Read the model definition and answer for the solid it produces. Units are mm, in the model's axes. A direction names the side the tool comes from. Coordinates: 2 decimals unless noted, no trailing zeros. Order: outer loops, then holes, each group sorted by start corner. A loop starts at its lowest first (then second) coordinate and runs counter-clockwise, first axis right, second up. Notation, with made-up numbers: (-28, 35) - (-9, 35) arc R16 ccw to (-9, 54) - close; hole circle Ø6 at (-34.75, 4). An arc over 180 degrees is marked (long way). Write item = value, one per line.
from build123d import *

# Parameters (mm, degrees)
SKETCH2_W                = 160
SKETCH2_H                = 130
BOSS_EXTRUDE1_DEPTH      = 6
SKETCH7_W                = 40
SKETCH7_H                = 40
CUT_EXTRUDE1_DEPTH       = 18
SKETCH9_R                = 2
CUT_EXTRUDE2_DEPTH       = 63
BOSS_EXTRUDE2_DEPTH      = 5
BOSS_EXTRUDE2_DEPTH_BACK = 10
SKETCH11_W               = 20
SKETCH11_H               = 15
CUT_EXTRUDE4_DEPTH       = 6
SKETCH13_R               = 2
CUT_EXTRUDE5_DEPTH       = 222
FILLET4_R                = 2
FILLET5_R                = 2
FILLET6_R                = 2


with BuildPart() as part:
    # Sketch2 → Boss-Extrude1 (new body)
    with BuildSketch(Plane(origin=(0, 0, 0), x_dir=(1, 0, 0), z_dir=(0, 1, 0))):
        Rectangle(SKETCH2_W, SKETCH2_H)
    extrude(amount=BOSS_EXTRUDE1_DEPTH)

    # Sketch7 → Cut-Extrude1 (cut)
    with BuildSketch(Plane(origin=(0, 6, 0), x_dir=(1, 0, 0), z_dir=(0, 1, 0))):
        with Locations((60, 45)):
            Rectangle(SKETCH7_W, SKETCH7_H)
    extrude(amount=-CUT_EXTRUDE1_DEPTH, mode=Mode.SUBTRACT)

    # Sketch9 → Cut-Extrude2 (cut)
    with BuildSketch(Plane.XY.offset(65)):
        with Locations((51.606058682, 2.978215898)):
            Circle(SKETCH9_R)
    extrude(amount=-CUT_EXTRUDE2_DEPTH, mode=Mode.SUBTRACT)

    # Sketch11 → Boss-Extrude2 (add, two sides: drawn at the far end of the back side and taken through both)
    with BuildSketch(Plane.XY.offset(65).offset(-BOSS_EXTRUDE2_DEPTH_BACK)):
        with Locations((51.606058682, 2.978215898)):
            Rectangle(SKETCH11_W, SKETCH11_H)
    extrude(amount=BOSS_EXTRUDE2_DEPTH + BOSS_EXTRUDE2_DEPTH_BACK)

    # Sketch12 → Cut-Extrude4 (cut)
    with BuildSketch(Plane.XY.offset(70)):
        Polygon((55.07279114, -3.020264415), (58.534261247, 2.981254118), (55.067528789, 8.979734431), (48.139326225, 8.976696212), (44.677856118, 2.975177679), (48.144588576, -3.023302634), align=None)
    extrude(amount=-CUT_EXTRUDE4_DEPTH, mode=Mode.SUBTRACT)

    # Sketch13 → Cut-Extrude5 (cut)
    with BuildSketch(Plane.XY.offset(64)):
        with Locations((51.606058682, 2.978215898)):
            Circle(SKETCH13_R)
    extrude(amount=-CUT_EXTRUDE5_DEPTH, mode=Mode.SUBTRACT)

    # Fillet4
    fillet4_edges = [part.edges().sort_by_distance(p)[0] for p in [
        (-80, 6, 0),
        (-80, 0, 0),
    ]]
    fillet(fillet4_edges, radius=FILLET4_R)

    # Fillet5
    # the kernel refuses this fillet: 2 mm, written as the material it takes off along each edge
    with BuildSketch(Plane(origin=(36.606058682, -4.521784102, 70), x_dir=(0, 0, -1), z_dir=(1, 0, 0)), Plane(origin=(36.606058682, -4.521784102, 55), x_dir=(0, 1, 0), z_dir=(1, 0, 0))) as fillet5_piece_1:
        with BuildLine():
            CenterArc((FILLET5_R, FILLET5_R), FILLET5_R, 180, 90)
            Line((0, FILLET5_R), (0, 0))
            Line((0, 0), (FILLET5_R, 0))
        make_face()
    extrude(amount=30, mode=Mode.SUBTRACT)
    with BuildSketch(Plane(origin=(61.606058682, -4.521784102, 50), x_dir=(0, 1, 0), z_dir=(0, 0, 1)), Plane(origin=(41.606058682, -4.521784102, 75), x_dir=(0, 1, 0), z_dir=(0, 0, -1))) as fillet5_piece_2:
        with BuildLine():
            CenterArc((FILLET5_R, FILLET5_R), FILLET5_R, 180, 90)
            Line((0, FILLET5_R), (0, 0))
            Line((0, 0), (FILLET5_R, 0))
        make_face()
    extrude(amount=25, mode=Mode.SUBTRACT)

    # Fillet6
    # the kernel refuses this fillet: 2 mm, written as the material it takes off along each edge
    with BuildSketch(Plane(origin=(66.606058682, 10.478215898, 70), x_dir=(0, 0, -1), z_dir=(-1, 0, 0))) as fillet6_piece_1:
        with BuildLine():
            CenterArc((FILLET6_R, FILLET6_R), FILLET6_R, 180, 90)
            Line((0, FILLET6_R), (0, 0))
            Line((0, 0), (FILLET6_R, 0))
        make_face()
    extrude(amount=30, mode=Mode.SUBTRACT)
    with BuildSketch(Plane(origin=(41.606058682, 10.478215898, 75), x_dir=(0, -1, 0), z_dir=(0, 0, -1)), Plane(origin=(61.606058682, 10.478215898, 50), x_dir=(0, -1, 0), z_dir=(0, 0, 1))) as fillet6_piece_2:
        with BuildLine():
            CenterArc((FILLET6_R, -FILLET6_R), FILLET6_R, 90, 90)
            Line((0, -FILLET6_R), (0, 0))
            Line((0, 0), (FILLET6_R, 0))
        make_face()
    extrude(amount=25, mode=Mode.SUBTRACT)
    with BuildSketch(Plane(origin=(66.606058682, 10.478215898, 55), x_dir=(0, 0, 1), z_dir=(-1, 0, 0))) as fillet6_piece_3:
        with BuildLine():
            CenterArc((FILLET6_R, -FILLET6_R), FILLET6_R, 90, 90)
            Line((0, -FILLET6_R), (0, 0))
            Line((0, 0), (FILLET6_R, 0))
        make_face()
    extrude(amount=30, mode=Mode.SUBTRACT)


solid = part.part
1) The part is cut by section C-C (x = -16.5). Determine the outline of the cut face in (y, z), and give its area (3 significant figures).
Returned:
outline = (0, -65) - (6, -65) - (6, 65) - (0, 65) - close
area = 780 mm^2
2) Determine the mould class of faces 5 (the face through (49.97, 4.4, 64)), 6 (the face through (40, 3, -45)), 7 (the face through (59, 3, 70)) for opening direction X: pulls with the +X half, pulls with the -X half, needs draft (parallel to the pull), parting line crosses it, or undercut.
Returned:
face_5 = undercut
face_6 = pulls with the +X half
face_7 = needs draft
3) Straight lines are drawn through the part: line 1 along Y through (x, z) = (-39, 27.5); line 2 along Z through (x, y) = (69.5, 0.5); line 3 along X through (y, z) = (3, -21.5). For each, find the intervals that lie inside material, in ascending order. Write a range as from..to.
Returned:
line_1 = 0..6
line_2 = -25..65
line_3 = -80..49.61, 53.61..80
4) The part is cut by section B-B (z = -29). Determine the outline of the cut face in (x, y).
Returned:
outline = (-80, 2) arc R2 ccw to (-78, 0) - (40, 0) - (40, 6) - (-78, 6) arc R2 ccw to (-80, 4) - close
5) The part is cut by section A-A (z = 23). Determine the outline of the cut face in (x, y), and give its area (3 significant figures).
Returned:
outline = (-80, 2) arc R2 ccw to (-78, 0) - (80, 0) - (80, 6) - (-78, 6) arc R2 ccw to (-80, 4) - close; hole circle Ø4 at (51.61, 2.98)
area = 946 mm^2
6) Flat-ended cylindrical pins translate along their axes: pin 1 Ø2 at (x, y) = (48.5, 7.5) entering from -Z; pin 2 Ø4.5 at (x, y) = (51.61, 2.98) entering from -Z; pin 3 Ø4 at (x, z) = (35.5, 36) entering from +Y; pin 4 Ø9 at (y, z) = (5.5, 64.5) entering from -X. Find the tip coordinate at first contact, or state that the pin passes through.
Returned:
pin_1 = 55
pin_2 = -25
pin_3 = 6
pin_4 = -80
7) For faces 1 (the face through (-20, 3, 65)), 2 (the face through (60, 3, -25)), 3 (the face through (56.825, 5.939, 67.042)), 4 (the face through (71, 3, 65)), determine the directions among +Z, -Z, +X, -X, +Y, -Y from which every point of the face is accessible in a straight line to the end or side of a thin tool.
Returned:
face_1 = +Z, -X, +Y, -Y
face_2 = -Z, +X, +Y, -Y
face_3 = +Z
face_4 = +Z, +X, +Y, -Y
